from build123d import *

# Parameters (mm, degrees)
F1_R = 13.49375
F3_R = 11.1125


with BuildPart() as f2:
    # F2: sweep along a path in F0
    with BuildLine(Plane.XZ) as f2_path:
        Line((0, 0), (0, 17.4625))
        ThreePointArc((0, 17.4625), (-4.6496798487, 28.6878201513), (-15.875, 33.3375))
        Line((-15.875, 33.3375), (-31.75, 33.3375))
    # F1 (on Top) → F2 (sweep)
    with BuildSketch(Plane.XY):
        Circle(F1_R)
    sweep(path=f2_path.line)

    # F4: sweep along a path in F0
    with BuildLine(Plane.XZ) as f4_path:
        Line((0, 0), (0, 17.4625))
        ThreePointArc((0, 17.4625), (-4.6496798487, 28.6878201513), (-15.875, 33.3375))
        Line((-15.875, 33.3375), (-31.75, 33.3375))
    # F3 (on face) → F4 (sweep, cut)
    with BuildSketch(Plane(origin=(0, 0, 0), x_dir=(1, 0, 0), z_dir=(0, 0, -1))):
        Circle(F3_R)
    sweep(path=f4_path.line, mode=Mode.SUBTRACT)


solid = f2.part
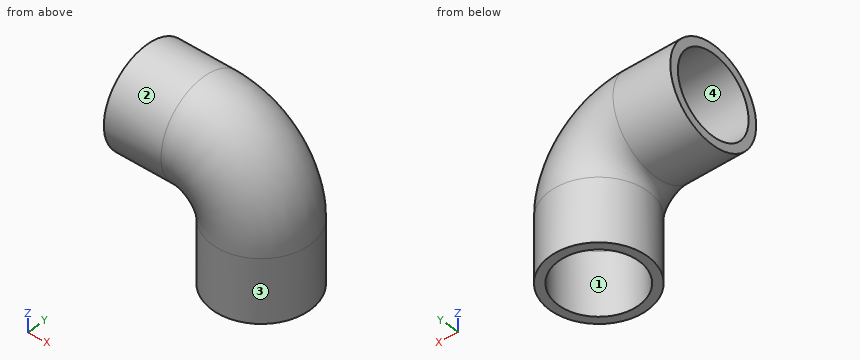
Check sheet for the modelled part. Datum: model origin and axes. Units: mm. Face numbers are marked on the shaded views. A direction names the side the tool comes from. Give positions to 0.01 mm unless a question says otherwise; leave off trailing zeros. Return JSON: item names as keys, results as strings. Group by question number.
1. Mould release check, pull along Y, two halves, no side actions. Record for the marked faces 3 and 4: released by +Y, released by -Y, zero draft, split by the parting line, or undercut.
2. Thickness scan on L1, parallel to Z at x = -20.5, y = -0.5; L2, parallel to Z at x = -20.25, y = 0 (3 decimals); L3, parallel to Y at x = 0, z = 6.25. Record the ranges inside material, lowest first.
3. Tool access check on the marked faces 1 and 2. Record the directions out of +Z, -Z, +X, -X, +Y, -Y that give a thin tool (end or side, any length) a straight path to the whole face; none if there is none.
4. Go/stop test with flat-tipped pins: pin 1 (5 mm diameter, centred on x = -5.5, z = 7.5, fed in from +Y); pin 2 (12 mm diameter, centred on x = -20.5, y = -7.5, fed in from +Z); pin 3 (5 mm diameter, centred on y = 0, z = 35.5, fed in from -X). Record where each tip stops, or that it passes through.
Return value:
{
 "1": {"face 3": "split by the parting line", "face 4": "undercut"},
 "2": {"L1": "19.85 to 22.24, 44.44 to 46.82", "L2": "19.844 to 22.225, 44.45 to 46.831", "L3": "-13.49 to -11.11, 11.11 to 13.49"},
 "3": {"face 1": "-Z", "face 2": "-X"},
 "4": {"pin 1": "y = 13.16", "pin 2": "z = 46.75", "pin 3": "x = 1.63"}
}
